from build123d import *

# Parameters (mm, degrees)
SKETCH021_W                    = 32
SKETCH021_H                    = 36
EXTRUDE019_DEPTH               = 1.5
SKETCH020_W                    = 36
SKETCH020_H                    = 36
EXTRUDE018_DEPTH               = 1
FUSION011_PLACEMENT_ANGLE      = 90
BASEFEATURE002_PLACEMENT_ANGLE = 90
POCKET002_DEPTH                = 5
PAD_DEPTH                      = 6.5
POCKET007_DEPTH                = 6.5
BODY003_PLACEMENT_ANGLE        = 90


with BuildPart() as extrude019:
    # Sketch021 (on Face6 of Extrude018) → Extrude019 (new body)
    with BuildSketch(Plane.XY.offset(1)):
        Rectangle(SKETCH021_W, SKETCH021_H)
    extrude(amount=EXTRUDE019_DEPTH)


with BuildPart() as body003:
    # Sketch020 → Extrude018 (new body)
    with BuildSketch(Plane.XY):
        Rectangle(SKETCH020_W, SKETCH020_H)
    extrude(amount=EXTRUDE018_DEPTH)

    # Fusion011: union Extrude019
    add(extrude019.part)


with BuildPart() as body003_1:
    # Fusion011 placement: moved
    add(body003.part.moved(Location((0, -17.5, 20))).rotate(Axis((0, -17.5, 20), (1, 0, 0)), FUSION011_PLACEMENT_ANGLE))


with BuildPart() as body003_2:
    # BaseFeature002 placement: moved
    add(body003_1.part.moved(Location((0, -20, -17.5))).rotate(Axis((0, -20, -17.5), (-1, 0, 0)), BASEFEATURE002_PLACEMENT_ANGLE))

    # Sketch026 (on Face8 of BaseFeature002) → Pocket002 (cut)
    with BuildSketch(Plane.XY.offset(2.5)):
        Polygon((0, 0), (0, 2.5), (5, 2.5), (5, -2.5), (-5, -2.5), (-5, 0), align=None)
    extrude(amount=-POCKET002_DEPTH, mode=Mode.SUBTRACT)

    # Sketch046 (on Face8 of Pocket002) → Pad (join)
    with BuildSketch(Plane.XY.offset(2.5)):
        Polygon((-2, 4.5), (7, 4.5), (7, -4.5), (-7, -4.5), (-7, 2), (-2, 2), align=None)
    extrude(amount=-PAD_DEPTH)

    # Sketch026 (on Face8 of BaseFeature002) → Pocket007 (cut)
    with BuildSketch(Plane.XY.offset(2.5)):
        Polygon((0, 0), (0, 2.5), (5, 2.5), (5, -2.5), (-5, -2.5), (-5, 0), align=None)
    extrude(amount=-POCKET007_DEPTH, mode=Mode.SUBTRACT)


with BuildPart() as body003_3:
    # Body003 placement: moved
    add(body003_2.part.moved(Location((0, -17.5, 20))).rotate(Axis((0, -17.5, 20), (1, 0, 0)), BODY003_PLACEMENT_ANGLE))


solid = body003_3.part
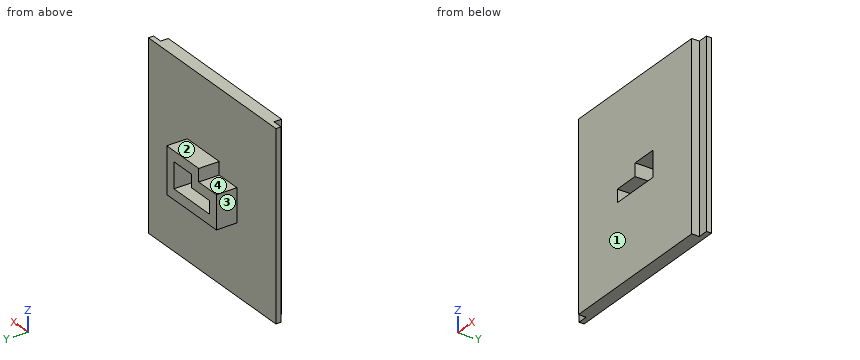
CAD build for the part. Positions are in the model's coordinates, mm. Face numbers are marked on the shaded views. A direction names the side the tool comes from. Round coordinates to 2 decimals unless told otherwise and drop trailing zeros. Loops run counter-clockwise (first coordinate to the right, second up) from the corner with the lowest first, then second, coordinate; pieces in that order, holes last.
(1) Which spindle directions (+Z, -Z, +X, -X, +Y, -Y) get a long thin tool onto all of the face, cutting with end or side? Do the marked faces 1, 2, 3 and 4. Say none if no direction does.
(2) Drop flat-ended pins along their axis: pin 1 (0.8 mm diameter, centred on y = -19.5, z = 20, fed in from +X); pin 2 (0.8 mm diameter, centred on y = -19.5, z = 21, fed in from -X); pin 3 (1.5 mm diameter, centred on x = 3.5, y = -15.5, fed in from -Z). Give the stop position or say it passes through.
(3) Wall check: line 1 along X through (y, z) = (-14, 18.5); line 2 along Z through (x, y) = (-1, -18.75); line 3 along X through (y, z) = (-18.25, 20.5). Give the ranges that are in metal, low to high.
(4) Cut at A-A (z = 21). Give the cut face in (x, y).
(5) Cut at C-C (x = -6.5). Give the cut face in (y, z), plus the area to 3 significant figures.
(6) Cut at B-B (y = -19.5). Give the cut face in (x, z).
(7) Cut at D-D (z = 12). Give the cut face in (x, y).
Findings below:
1. face 1: +Z, -Z, +X, -X, -Y
1. face 2: +Z, +X, -X, +Y
1. face 3: +Z, -Z, -X, +Y
1. face 4: +Z, -X, +Y
2. pin 1: stops at x = 16
2. pin 2: stops at x = -16
2. pin 3: stops at z = 15.5
3. line 1: x = -7 to -5, 5 to 7
3. line 2: z = 2 to 17.5, 20 to 38
3. line 3: x = -18 to 0, 5 to 18
4. outline: (-18, -18.5) - (-16, -18.5) - (-16, -20) - (0, -20) - (0, -13.5) - (-7, -13.5) - (-7, -17.5) - (-18, -17.5) - close; (5, -20) - (16, -20) - (16, -18.5) - (18, -18.5) - (18, -17.5) - (7, -17.5) - (7, -13.5) - (5, -13.5) - close
5. outline: (-20, 2) - (-17.5, 2) - (-17.5, 15.5) - (-13.5, 15.5) - (-13.5, 22) - (-17.5, 22) - (-17.5, 38) - (-20, 38) - close
5. area: 116 mm2
6. outline: (-16, 2) - (16, 2) - (16, 38) - (-16, 38) - close; hole (-5, 17.5) - (5, 17.5) - (5, 22.5) - (0, 22.5) - (0, 20) - (-5, 20) - close
7. outline: (-18, -18.5) - (-16, -18.5) - (-16, -20) - (16, -20) - (16, -18.5) - (18, -18.5) - (18, -17.5) - (-18, -17.5) - close
